The model under review builds one solid part; all positions refer to its coordinate system, in mm. A direction names the side the tool comes from. Coordinates: 2 decimals unless noted, no trailing zeros. Order: outer loops, then holes, each group sorted by start corner. A loop starts at its lowest first (then second) coordinate and runs counter-clockwise, first axis right, second up. Notation, with made-up numbers: (56, 20) - (68, 20) arc R15 ccw to (68, 46) - close; hole circle Ø9 at (-0.75, 26). An arc over 180 degrees is marked (long way). Answer in a Markdown table with one row per item.
```python
from build123d import *

# Parameters (mm, degrees)
F0_W         = 100
F0_H         = 36
F1_DEPTH     = 20
F2_W         = 20
F2_H         = 20
F3_DEPTH     = 10
F4_R         = 9.99999
F5_T4_DEPTH  = 200.6036926139
F5_T10_DEPTH = 200.6036926139
F5_T16_DEPTH = 200.6036926139
F5_T23_DEPTH = 200.6036926139
F5_T29_DEPTH = 200.6036926139
F6_R         = 6
F7_DEPTH     = 10.001
F8_T4_DEPTH  = 200.6036926139
F8_T10_DEPTH = 200.6036926139
F8_T16_DEPTH = 200.6036926139
F8_T23_DEPTH = 200.6036926139
F8_T29_DEPTH = 200.6036926139
F9_R         = 27
F10_DEPTH    = 10
F11_R        = 19
F12_DEPTH    = 10
F13_R        = 19
F14_DEPTH    = 20
F15_R        = 10
F16_DEPTH    = 20.001


# Not quite as in the source:
# - a fillet or chamfer that OpenCascade refuses, or shapes differently, is made with other operations: its cross-section is extruded or revolved along the edge and cut away or added
# - a fillet or chamfer is up to 0.001 mm smaller than in the source, because OpenCascade refuses the exact size
# - a pattern or mirror of a feature is missing from the dataset's text; its kind, count and spacing are read off the source's solid


with BuildPart() as f1:
    # F0 (on Right) → F1 (new body, symmetric)
    with BuildSketch(Plane.YZ):
        Rectangle(F0_W, F0_H)
    extrude(amount=F1_DEPTH, both=True)

    # F2 (on face) → F3 (join)
    with BuildSketch(Plane(origin=(0, 0, -18), x_dir=(1, 0, 0), z_dir=(0, 0, -1))):
        with Locations((0, 60)):
            Rectangle(F2_W, F2_H)
    f3 = extrude(amount=-F3_DEPTH)

    # F3_copies: F3 across plane
    add(f3.mirror(Plane.ZX.offset(-3e-06)))

    # F4 (radius 10 in the source; OpenCascade refuses exactly that, so slightly less here)
    f4_edges = [f1.edges().sort_by_distance(p)[0] for p in [
        (10, -70, -13),
        (-10, -70, -13),
        (-10, 69.999994, -13),
        (10, 69.999994, -13),
    ]]
    fillet(f4_edges, radius=F4_R)

    # F5: chamfer of 15 x 31 on 1 edges, made by hand


with BuildPart() as f5_tool2:
    # F5_s3 → F5_t4 (new body)
    with BuildSketch(Plane.YZ.offset(-100.301846307)):
        Polygon((-50, -13), (-35, 18), (-50, 18), align=None)
    extrude(amount=F5_T4_DEPTH)

    split(bisect_by=Plane.XY.offset(-8), keep=Keep.BOTTOM)

    split(bisect_by=Plane.YZ.offset(-10), keep=Keep.BOTTOM)


with BuildPart() as f1_1:
    add(f1.part)

    # F5_t1: cut F5_tool2
    add(f5_tool2.part, mode=Mode.SUBTRACT)


with BuildPart() as f5_tool8:
    # F5_s9 → F5_t10 (new body)
    with BuildSketch(Plane.YZ.offset(-100.301846307)):
        Polygon((-50, -13), (-35, 18), (-50, 18), align=None)
    extrude(amount=F5_T10_DEPTH)

    split(bisect_by=Plane.XY.offset(-8), keep=Keep.TOP)

    split(bisect_by=Plane.YZ.offset(-10), keep=Keep.BOTTOM)


with BuildPart() as f1_2:
    add(f1_1.part)

    # F5_t7: cut F5_tool8
    add(f5_tool8.part, mode=Mode.SUBTRACT)


with BuildPart() as f5_tool14:
    # F5_s15 → F5_t16 (new body)
    with BuildSketch(Plane.YZ.offset(-100.301846307)):
        Polygon((-50, -13), (-35, 18), (-50, 18), align=None)
    extrude(amount=F5_T16_DEPTH)

    split(bisect_by=Plane.YZ.offset(10), keep=Keep.BOTTOM)

    split(bisect_by=Plane.XY.offset(-8), keep=Keep.TOP)

    split(bisect_by=Plane.YZ.offset(-10), keep=Keep.TOP)


with BuildPart() as f1_3:
    add(f1_2.part)

    # F5_t13: cut F5_tool14
    add(f5_tool14.part, mode=Mode.SUBTRACT)


with BuildPart() as f5_tool21:
    # F5_s22 → F5_t23 (new body)
    with BuildSketch(Plane.YZ.offset(-100.301846307)):
        Polygon((-50, -13), (-35, 18), (-50, 18), align=None)
    extrude(amount=F5_T23_DEPTH)

    split(bisect_by=Plane.YZ.offset(10), keep=Keep.TOP)

    split(bisect_by=Plane.XY.offset(-8), keep=Keep.BOTTOM)


with BuildPart() as f1_4:
    add(f1_3.part)

    # F5_t20: cut F5_tool21
    add(f5_tool21.part, mode=Mode.SUBTRACT)


with BuildPart() as f5_tool27:
    # F5_s28 → F5_t29 (new body)
    with BuildSketch(Plane.YZ.offset(-100.301846307)):
        Polygon((-50, -13), (-35, 18), (-50, 18), align=None)
    extrude(amount=F5_T29_DEPTH)

    split(bisect_by=Plane.YZ.offset(10), keep=Keep.TOP)

    split(bisect_by=Plane.XY.offset(-8), keep=Keep.TOP)


with BuildPart() as f1_5:
    add(f1_4.part)

    # F5_t26: cut F5_tool27
    add(f5_tool27.part, mode=Mode.SUBTRACT)

    # F6 (on face) → F7 (cut, through all)
    with BuildSketch(Plane.XY.offset(-8)):
        with Locations((0, -60)):
            Circle(F6_R)
    f7 = extrude(amount=-F7_DEPTH, mode=Mode.SUBTRACT)

    # F7_copies: F7 across plane
    add(f7.mirror(Plane.ZX), mode=Mode.SUBTRACT)

    # F8: chamfer of 15 x 31 on 1 edges, made by hand


with BuildPart() as f8_tool2:
    # F8_s3 → F8_t4 (new body)
    with BuildSketch(Plane.YZ.offset(100.301846307)):
        Polygon((50, -13), (35, 18), (50, 18), align=None)
    extrude(amount=-F8_T4_DEPTH)

    split(bisect_by=Plane.XY.offset(-8), keep=Keep.BOTTOM)

    split(bisect_by=Plane.YZ.offset(10), keep=Keep.TOP)


with BuildPart() as f1_6:
    add(f1_5.part)

    # F8_t1: cut F8_tool2
    add(f8_tool2.part, mode=Mode.SUBTRACT)


with BuildPart() as f8_tool8:
    # F8_s9 → F8_t10 (new body)
    with BuildSketch(Plane.YZ.offset(100.301846307)):
        Polygon((50, -13), (35, 18), (50, 18), align=None)
    extrude(amount=-F8_T10_DEPTH)

    split(bisect_by=Plane.XY.offset(-8), keep=Keep.TOP)

    split(bisect_by=Plane.YZ.offset(10), keep=Keep.TOP)


with BuildPart() as f1_7:
    add(f1_6.part)

    # F8_t7: cut F8_tool8
    add(f8_tool8.part, mode=Mode.SUBTRACT)


with BuildPart() as f8_tool14:
    # F8_s15 → F8_t16 (new body)
    with BuildSketch(Plane.YZ.offset(100.301846307)):
        Polygon((50, -13), (35, 18), (50, 18), align=None)
    extrude(amount=-F8_T16_DEPTH)

    split(bisect_by=Plane.YZ.offset(-10), keep=Keep.TOP)

    split(bisect_by=Plane.XY.offset(-8), keep=Keep.TOP)

    split(bisect_by=Plane.YZ.offset(10), keep=Keep.BOTTOM)


with BuildPart() as f1_8:
    add(f1_7.part)

    # F8_t13: cut F8_tool14
    add(f8_tool14.part, mode=Mode.SUBTRACT)


with BuildPart() as f8_tool21:
    # F8_s22 → F8_t23 (new body)
    with BuildSketch(Plane.YZ.offset(100.301846307)):
        Polygon((50, -13), (35, 18), (50, 18), align=None)
    extrude(amount=-F8_T23_DEPTH)

    split(bisect_by=Plane.YZ.offset(-10), keep=Keep.BOTTOM)

    split(bisect_by=Plane.XY.offset(-8), keep=Keep.BOTTOM)


with BuildPart() as f1_9:
    add(f1_8.part)

    # F8_t20: cut F8_tool21
    add(f8_tool21.part, mode=Mode.SUBTRACT)


with BuildPart() as f8_tool27:
    # F8_s28 → F8_t29 (new body)
    with BuildSketch(Plane.YZ.offset(100.301846307)):
        Polygon((50, -13), (35, 18), (50, 18), align=None)
    extrude(amount=-F8_T29_DEPTH)

    split(bisect_by=Plane.YZ.offset(-10), keep=Keep.BOTTOM)

    split(bisect_by=Plane.XY.offset(-8), keep=Keep.TOP)


with BuildPart() as f1_10:
    add(f1_9.part)

    # F8_t26: cut F8_tool27
    add(f8_tool27.part, mode=Mode.SUBTRACT)

    # F9 (on face) → F10 (cut)
    with BuildSketch(Plane.YZ.offset(20)):
        with Locations((0, 18)):
            Circle(F9_R)
    extrude(amount=-F10_DEPTH, mode=Mode.SUBTRACT)

    # F11 (on face) → F12 (cut)
    with BuildSketch(Plane.YZ.offset(10)):
        with Locations((0, 18)):
            Circle(F11_R)
    extrude(amount=-F12_DEPTH, mode=Mode.SUBTRACT)

    # F13 (on face) → F14 (join)
    with BuildSketch(Plane.YZ):
        with Locations((0, 18)):
            Circle(F13_R)
    extrude(amount=-F14_DEPTH)

    # F15 (on face) → F16 (cut, through all)
    with BuildSketch(Plane.YZ):
        with Locations((0, 18)):
            Circle(F15_R)
    extrude(amount=-F16_DEPTH, mode=Mode.SUBTRACT)


solid = f1_10.part
```
Item 1: We need section D-D, the plane z = -3.5. Write out the cut boundary in (x, y), then the cut area to 3 significant figures.
Check values:
| item | result |
|---|---|
| outline | (-20, -45.4) - (20, -45.4) - (20, -16.33) - (10, -16.33) - (10, 16.33) - (20, 16.33) - (20, 45.4) - (-20, 45.4) - close |
| area | 3,310 mm^2 |
Item 2: We need section B-B, the plane x = 4. Write out the cut boundary in (y, z).
Check values:
| item | result |
|---|---|
| outline | (-69.17, -18) - (-64.47, -18) - (-64.47, -8) - (-69.17, -8) - close; (-55.53, -18) - (55.53, -18) - (55.53, -8) - (47.58, -8) - (35, 18) - (19, 18) arc R19 cw to (-19, 18) - (-35, 18) - (-47.58, -8) - (-55.53, -8) - close; (64.47, -18) - (69.17, -18) - (69.17, -8) - (64.47, -8) - close |
Item 3: To check wall thickness, follow line 1 (Z direction, x = -18, y = 22.5); line 2 (Z direction, x = 5, y = 55.5); line 3 (Z direction, x = -10, y = 0). State the ranges of each line that lie inside material, in increasing order. Write a range as from..to.
Check values:
| item | result |
|---|---|
| line 1 | -18..18 |
| line 2 | -18..-8 |
| line 3 | -18..8, 28..37 |
Item 4: Clearance check with flat-ended pins moving along their axes: pin 1 Ø6 at (x, y) = (-3.5, -62.5) entering from +Z; pin 2 Ø11 at (x, y) = (0, -60) entering from +Z; pin 3 Ø21.5 at (y, z) = (-6.5, 6) entering from +X; pin 4 Ø3 at (y, z) = (52.5, -11.5) entering from -X. State where each tip first meets the part, or that it passes through.
Check values:
| item | result |
|---|---|
| pin 1 | z = -8 |
| pin 2 | through |
| pin 3 | x = 10 |
| pin 4 | x = -10 |
Item 5: We need section A-A, the plane y = 0. Write out the cut boundary in (x, z).
Check values:
| item | result |
|---|---|
| outline | (-20, -18) - (20, -18) - (20, -9) - (10, -9) - (10, -1) - (0, -1) - (0, 8) - (-20, 8) - close; (-20, 28) - (0, 28) - (0, 37) - (-20, 37) - close |
Item 6: Mouldability with a two-part tool opening along Y and no side actions: class faces 4 (the face through (-2, 54, -8)), 5 (the face through (0, 8, 10)), 6 (the face through (6.99, 67.15, -12.93)), 7 (the face through (-10, 0, 37)) as +Y half, -Y half, draft (parallel to the pull), parting line (faces both ways), or undercut.
Check values:
| item | result |
|---|---|
| face 4 | draft |
| face 5 | undercut |
| face 6 | +Y half |
| face 7 | parting line |
Item 7: We need section C-C, the plane z = 14. Write out the cut boundary in (x, y), then the cut area to 3 significant figures.
Check values:
| item | result |
|---|---|
| outline | (-20, -36.94) - (20, -36.94) - (20, -26.7) - (10, -26.7) - (10, -18.57) - (0, -18.57) - (0, -9.17) - (-20, -9.17) - close; (-20, 9.17) - (0, 9.17) - (0, 18.57) - (10, 18.57) - (10, 26.7) - (20, 26.7) - (20, 36.94) - (-20, 36.94) - close |
| area | 1,680 mm^2 |
Item 8: Tool access review of faces 1 (the face through (-15, 50, -16)), 2 (the face through (0, 27, 18)), 3 (the face through (15.07, -0.594, -8.993)): name each direction out of +Z, -Z, +X, -X, +Y, -Y from which nothing blocks a thin tool from reaching the whole face with its end or side.
Check values:
| item | result |
|---|---|
| face 1 | +Z, -Z, -X, +Y |
| face 2 | +Z, +X, -X, +Y |
| face 3 | +Z, +X |
